Geometry: final body of the model. Coordinates: model frame, mm. A direction names the side the tool comes from. Give positions to 0.01 mm unless a question says otherwise; leave off trailing zeros. Loops run counter-clockwise (first coordinate to the right, second up) from the corner with the lowest first, then second, coordinate; pieces in that order, holes last.
1. Section A-A, the plane y = 9. Output: boundary loops of the cut face in (x, z) (3 decimals).
2. Material intervals for line 1 along Z through (x, y) = (-140.5, 20.75) (3 decimals); line 2 along Z through (x, y) = (130, 17.25), sorted ascending.
3. Section B-B, the plane x = 23.5. Output: boundary loops of the cut face in (y, z).
4. Access query for faces 1 (the face through (-78, 13, 3.175)), 2 (the face through (-78, 13, 0)). Directions: +Z, -Z, +X, -X, +Y, -Y. A direction counts if a zero-diameter tool reaches every point of the face in a straight line with its end or side. Return the directions, or none.
5. First-contact query: P1, Ø1, axis at x = 92, y = 11, coming from the -Z side; P2, Ø3, axis at x = 35.5, z = 10.5, coming from the -Y side; P3, Ø10, axis at x = -37.5, y = 16.5, coming from the +Z side (3 decimals). Flat tips, straight axial feed; report the tip coordinate or a pass-through.
6. Section C-C, the plane z = 10.5. Output: boundary loops of the cut face in (x, y), then the cut area to 3 significant figures.
Autodesk Inventor part; units mm, degrees
ref_plane "YZ Plane" through (0, 0, 0) normal (1, 0, 0) x (0, 1, 0)
ref_plane "XZ Plane" through (0, 0, 0) normal (0, 1, 0) x (-1, 0, 0)
ref_plane "XY Plane" through (0, 0, 0) normal (0, 0, 1) x (1, 0, 0)
sketch "Sketch1" plane through (0, 0, 0) normal (0, 0, 1) x (1, 0, 0)
  line L0 (0, 0) -> (-154.1018, 0)
  line L1 (-154.1018, 0) -> (-154.1018, 25.4)
  line L2 (-154.1018, 25.4) -> (0, 25.4)
  line L3 (0, 25.4) -> (0, 0)
  dimension "d0" = 154.1018
  dimension "d1" = 25.4
extrude "Plate1" add sketch "Sketch1" along normal blind 3.175
sketch "Sketch2" plane through (0, 0, 3.175) normal (0, 0, 1) x (1, 0, 0)
  line L0 (-154.1018, 0) -> (-154.1018, 25.4)
  line L1 (0, 0) -> (-154.1018, 0)
  line L2 (0, 25.4) -> (0, 0)
  line L3 (-154.1018, 25.4) -> (0, 25.4)
  line L4 (-154.1018, 25.4) -> (-1.7018, 25.4)
  line L5 (-1.7018, 25.4) -> (-77.0509, 0)
  dimension "d3" = 152.4
sketch "Sketch3" plane through (-0.9315, 25.4, 3.0353) normal (0.293373, 0, -0.9559981) x (0, 1, 0)
  line L0 (-25.4, 0) -> (0, 0)
  line L1 (0, 0) -> (0, 152.4)
  line L2 (0, 152.4) -> (-25.4, 152.4)
  line L3 (-25.4, 152.4) -> (-25.4, 0)
edge flange "Flange1" height 152.4 angle 17.06 thickness 3.175 bend radius 1.27 thickness toward (0.293373, 0, -0.9559981) relief straight relief width 3.175 relief depth 1.5875 edges at (0, 12.7, 3.175) wall of the first edge with corners at (-0.9315, 0, 3.0353) (-0.9315, 25.4, 3.0353) (144.7626, 25.4, 47.7453) (144.7626, 0, 47.7453)
bend "Bend1"
corner "Corner1"
equation "\"d4\" = BendReliefWidth"
equation "\"d5\" = BendReliefDepth"
equation "\"d6\" = MinimumRemnant"
equation "\"d7\" = BendRadius"
equation "\"d11\" = CornerReliefSize"
equation "\"d12\" = GapSize"
equation "\"d13\" = JacobiRadiusSize"
equation "\"BendRadius\" = Thickness"
equation "\"BendReliefWidth\" = Thickness"
equation "\"BendReliefDepth\" = 0.5 * Thickness"
equation "\"CornerReliefSize\" = 4 * Thickness"
equation "\"MinimumRemnant\" = 2 * Thickness"
equation "\"TransitionRadius\" = BendRadius"
equation "\"JacobiRadiusSize\" = Thickness"
equation "\"GapSize\" = Thickness"
equation "\"d2\" = BendRadius"
properties part number "bent plough"
Answers below:
1. outline: (-154.102, 0) - (-0.667, 0) arc R4.445 ccw to (0.637, 0.196) - (145.694, 44.71) - (144.763, 47.745) - (-0.294, 3.231) arc R1.27 cw to (-0.667, 3.175) - (-154.102, 3.175) - close
2. line 1: z = 0 to 3.175
2. line 2: z = 39.89 to 43.22
3. outline: (0, 7.21) - (25.4, 7.21) - (25.4, 10.53) - (0, 10.53) - close
4. face 1: +Z, -X, +Y, -Y
4. face 2: -Z, +X, -X, +Y, -Y
5. P1: stops at z = 28.08
5. P2: stops at y = 0
5. P3: stops at z = 3.175
6. outline: (23.39, 0) - (34.22, 0) - (34.22, 25.4) - (23.39, 25.4) - close
6. area: 275 mm2
